Autodesk Inventor part; units mm, degrees
ref_plane "YZ Plane" through (0, 0, 0) normal (1, 0, 0) x (0, 1, 0)
ref_plane "XZ Plane" through (0, 0, 0) normal (0, 1, 0) x (-1, 0, 0)
ref_plane "XY Plane" through (0, 0, 0) normal (0, 0, 1) x (1, 0, 0)
sketch "Sketch1" plane through (0, 0, 0) normal (0, 0, 1) x (1, 0, 0)
  circle A0 centre (0, 0) radius 36.5
  circle A1 centre (0, 0) radius 32.5
  circle A2 centre (0, 0) radius 16
  circle A3 centre (0, 0) radius 2.7
  line L0 (0, 0) -> (-8.4116, 31.3926)
  line L1 (0, 0) -> (8.4116, 31.3926)
  line L2 (0, 0) -> (0, 4.5704)
  line L3 (0, 0) -> (-32.4555, 1.7009)
  line L4 (0, 0) -> (-27.2568, 17.7008)
  line L5 (0, 0) -> (-11.647, -30.3414)
  line L6 (0, 0) -> (-25.2572, -20.4529)
  line L7 (0, 0) -> (25.2572, -20.4529)
  line L8 (0, 0) -> (11.647, -30.3414)
  line L9 (0, 0) -> (27.2568, 17.7008)
  line L10 (0, 0) -> (32.4555, 1.7009)
  point P0 (4.1411, 15.4548)
  point P1 (13.4187, 8.7142)
  point P2 (-4.1411, 15.4548)
  point P3 (-13.4187, 8.7142)
  point P4 (12.4343, -10.0691)
  point P5 (15.9781, 0.8374)
  point P6 (-5.7339, -14.9373)
  point P7 (5.7339, -14.9373)
  point P8 (-15.9781, 0.8374)
  point P9 (-12.4343, -10.0691)
  dimension "d0" = 73
  dimension "d1" = 65
  dimension "d2" = 5.4
  dimension "d3" = 32
  dimension "d4" = 15
  dimension "d5" = 15
  dimension "d8" = 360
extrude "Extrusion1" add sketch "Sketch1" along normal blind 3 contours A0 | L10 A2 L9 A1 | A1 L8 A2 L7 | L10 A3 L9 A2 | A2 L7 A3 L10 | A2 L8 A3 L7 | L1 A2 L0 A1 | L9 A3 L1 A2 | A1 L6 A2 L5 | A2 L5 A3 L8 | L1 A3 L0 A2 | A2 L6 A3 L5 | L4 A2 L3 A1 | L0 A3 L4 A2 | L3 A2 L4 A3 | A3 L6 A2 L3
fillet "Fillet1" radius 10 10 edges at (8.4116, 31.3926, 1.5) (-27.2568, 17.7008, 1.5) (-25.2572, -20.4529, 1.5) (11.647, -30.3414, 1.5) (32.4555, 1.7009, 1.5) (-15.9781, 0.8374, 1.5) (-4.1411, 15.4548, 1.5) (13.4187, 8.7142, 1.5) (12.4343, -10.0691, 1.5) (-5.7339, -14.9373, 1.5)
sketch "Sketch2" plane through (0, 0, 3) normal (0, 0, 1) x (1, 0, 0)
  circle A0 centre (0, 12.0208) radius 1.7
  circle A1 centre (-12.0208, 0) radius 1.7
  circle A2 centre (0, -12.0208) radius 1.7
  circle A3 centre (12.0208, 0) radius 1.7
  line L0 (0, 12.0208) -> (-12.0208, 0)
  line L1 (-12.0208, 0) -> (0, -12.0208)
  line L2 (0, -12.0208) -> (12.0208, 0)
  line L3 (12.0208, 0) -> (0, 12.0208)
  point P0 (0, 0)
  dimension "d13" = 17
  dimension "d14" = 17
  dimension "d15" = 3.4
  dimension "d16" = 3.4
  dimension "d17" = 3.4
  dimension "d18" = 3.4
extrude "Extrusion2" cut sketch "Sketch2" against normal blind 3 contours A0 L3 L0 | L0 L3 A0 | L0 L1 A1 | A1 L1 L0 | L3 L2 A3 | A3 L2 L3 | L1 L2 A2 | A2 L2 L1
properties part number "Wheel_2D_1"
Design review of the part built by this model. Coordinates are the model's own, in mm. Give positions to 0.01 mm unless a question says otherwise; leave off trailing zeros. Order: outer loops, then holes, each group sorted by start corner. A loop starts at its lowest first (then second) coordinate and runs counter-clockwise, first axis right, second up. Notation, with made-up numbers: (70.5, 43) -> (95.5, 43) arc R29 ccw to (95.5, 79) -> close; hole circle Ø8 at (74, 49.25). An arc over 180 degrees is marked (long way). Write each question's results on one line, items separated by ' | '. Start each with the question number.
Q1. Add section D-D on x = -28. Give the boundary of the cut face in (y, z).
Q2. For pin 1 (2 mm diameter, centred on x = 12.02, y = 0, fed in from -Z); pin 2 (1.5 mm diameter, centred on x = -11, z = 1, fed in from -Y), all flat-tipped, find the tip position at first contact; note any pin that passes through.
Q3. Add section C-C on x = 11.5. Give the boundary of the cut face in (y, z).
Q4. Add section B-B on y = 30. Give the boundary of the cut face in (x, z).
Q5. Add section A-A on y = 21. Give the boundary of the cut face in (x, z).
Q6. Wall thickness on L1, parallel to Y at x = -13, z = 0.4; L2, parallel to Y at x = 0, z = 1.7; L3, parallel to X at y = -8, z = 1.75: over which ranges is each line inside the solid? List them lowest first. Write a range as from..to.
Q7. Mouldability with a two-part tool opening along Y and no side actions: class faces 1 (the flat face through (-1, -8, 3)), 2 (the cylindrical face through (15.373, -10.229, 1.521)) as +Y half, -Y half, draft (parallel to the pull), parting line (faces both ways), or undercut.
Found:
1) outline: (-23.41, 0) -> (-12.88, 0) -> (-12.88, 3) -> (-23.41, 3) -> close; (1.47, 0) -> (23.41, 0) -> (23.41, 3) -> (1.47, 3) -> close
2) pin 1: passes through | pin 2: stops at y = -35.03
3) outline: (-34.64, 0) -> (-1.62, 0) -> (-1.62, 3) -> (-34.64, 3) -> close; (1.62, 0) -> (11.98, 0) -> (11.98, 3) -> (1.62, 3) -> close; (26.29, 0) -> (34.64, 0) -> (34.64, 3) -> (26.29, 3) -> close
4) outline: (-20.79, 0) -> (-12.5, 0) -> (-12.5, 3) -> (-20.79, 3) -> close; (-8.04, 0) -> (20.79, 0) -> (20.79, 3) -> (-8.04, 3) -> close
5) outline: (-29.85, 0) -> (-21.32, 0) -> (-21.32, 3) -> (-29.85, 3) -> close; (-5.88, 0) -> (5.76, 0) -> (5.76, 3) -> (-5.88, 3) -> close; (24.8, 0) -> (29.85, 0) -> (29.85, 3) -> (24.8, 3) -> close
6) L1: y = -34.11..-10.53, -9.33..-1.39, 1.39..9.33, 29.79..34.11 | L2: y = -36.5..-32.17, -16.02..-13.72, -10.32..-2.7, 2.7..10.32, 13.72..36.5 | L3: x = -35.61..-31.47, -13.86..14.97, 30.61..35.61
7) face 1: draft | face 2: undercut
